Answer from the drawing. Dimensions are ordinates in mm from the lowest x, y and z of the part. Give positions to 0.01 mm unless a question says otherwise; leave off trailing zeros. Write each loop counter-clockwise with the first axis right and the second up, starting at its lowest first coordinate (ties: lowest second). Pieces come first, ordered by that corner, then holes. Notation, with made-up numbers: (-13.5, 26.25) -> (-0.5, 26.25) arc R26 cw to (-0.5, 53.25) -> close; hole circle Ø5 at (67.5, 67). An arc over 180 degrees is marked (long way). Use a Markdown table: item, result. Add a question column.
Q1. Consider line 1 (Z direction, x = 103, y = 1.5) (1 decimal); line 2 (X direction, y = 2, z = 132.5); line 3 (X direction, y = 2.5, z = 114.5). Determine where each line is inside the solid, lowest interval first.
Q2. Section A-A, the plane x = 101.6 is taken. Give the vertices of the cut face in (y, z).
Q3. Each of these flat-tipped pins is pushed along its axis until it touches: pin 1 Ø4 at (x, z) = (186.27, 134.44) entering from -Y; pin 2 Ø4 at (x, z) = (66, 174) entering from -Y. Where does it stop, or does it pass through?
Q4. Section B-B, the plane y = 2 is taken. Give the vertices of the cut face in (x, z).
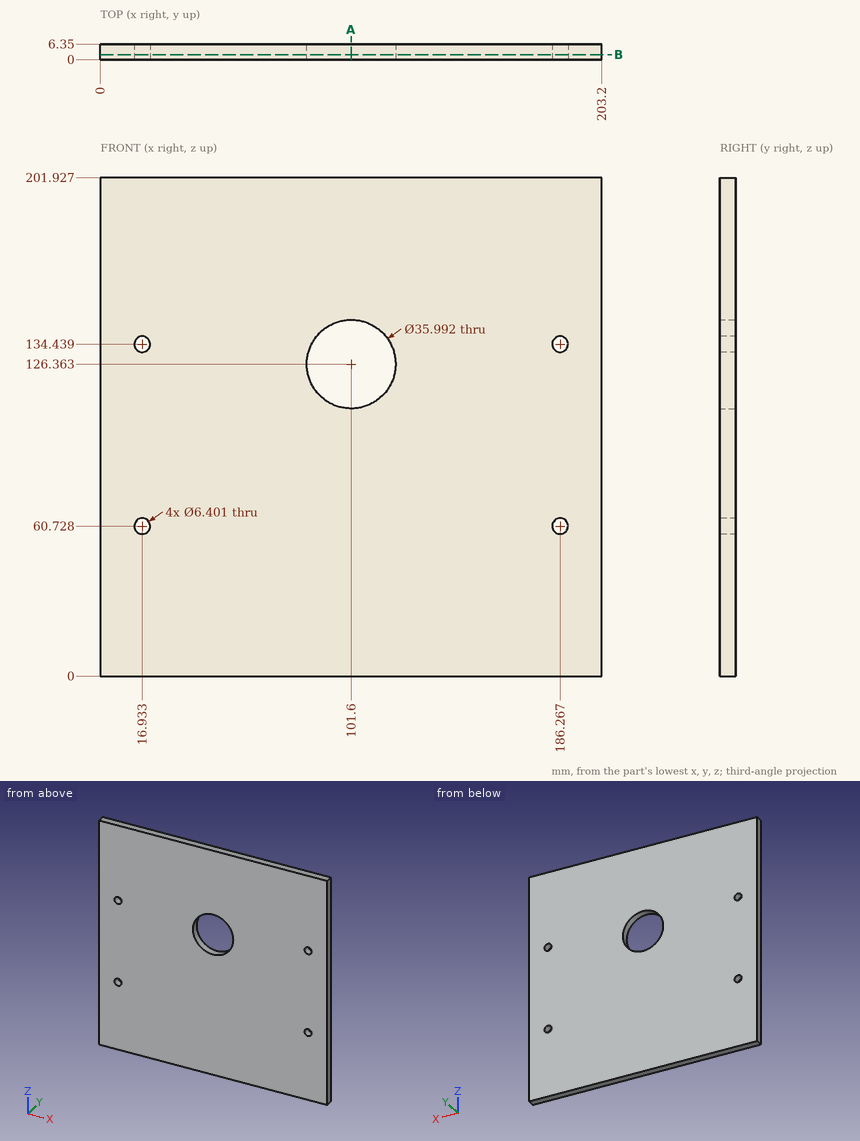
Result set:
| question | item | result |
|---|---|---|
| 1 | line 1 | z = 0 to 108.4, 144.3 to 201.9 |
| 1 | line 2 | x = 0 to 14.39, 19.48 to 84.68, 118.52 to 183.72, 188.81 to 203.2 |
| 1 | line 3 | x = 0 to 88.07, 115.13 to 203.2 |
| 2 | outline | (0, 0) -> (6.35, 0) -> (6.35, 108.37) -> (0, 108.37) -> close; (0, 144.36) -> (6.35, 144.36) -> (6.35, 201.93) -> (0, 201.93) -> close |
| 3 | pin 1 | passes through |
| 3 | pin 2 | stops at y = 0 |
| 4 | outline | (0, 0) -> (203.2, 0) -> (203.2, 201.93) -> (0, 201.93) -> close; hole circle Ø6.4 at (16.93, 60.73); hole circle Ø6.4 at (16.93, 134.44); hole circle Ø35.99 at (101.6, 126.36); hole circle Ø6.4 at (186.27, 60.73); hole circle Ø6.4 at (186.27, 134.44) |
